from build123d import *

# Parameters (mm, degrees)
F0_W      = 42
F0_H      = 38.608
F1_DEPTH  = 7.493
F2_R      = 1.905
F3_DEPTH  = 7.494
F4_R      = 1.905
F5_DEPTH  = 25.4
F6_R      = 3.302
F6_R_2    = 1.905
F7_DEPTH  = 3.048
F8_R      = 3.5
F9_DEPTH  = 7.494
F10_R     = 12
F11_DEPTH = 3
F13_DEPTH = 3.81


with BuildPart() as f1:
    # F0 (on Top) → F1 (new body)
    with BuildSketch(Plane.XY):
        Rectangle(F0_W, F0_H)
    extrude(amount=F1_DEPTH)

    # F2 (on face) → F3 (cut, through all)
    with BuildSketch(Plane.XY.offset(7.493)):
        with Locations((-14.8492424049, 14.8492424049)):
            Circle(F2_R)
        with Locations((14.8492424049, -14.8492424049)):
            Circle(F2_R)
    extrude(amount=-F3_DEPTH, mode=Mode.SUBTRACT)

    # F4 (on face) → F5 (cut)
    with BuildSketch(Plane.XY.offset(7.493)):
        with Locations((15.5, 15.5)):
            Circle(F4_R)
        with Locations((-15.5, -15.5)):
            Circle(F4_R)
    extrude(amount=-F5_DEPTH, mode=Mode.SUBTRACT)

    # F6 (on face) → F7 (cut)
    with BuildSketch(Plane.XY.offset(7.493)):
        with Locations((15.5, 15.5)):
            Circle(F6_R)
        with Locations((15.5, 15.5)):
            Circle(F6_R_2, mode=Mode.SUBTRACT)
        with Locations((-15.5, -15.5)):
            Circle(F6_R)
        with Locations((-15.5, -15.5)):
            Circle(F6_R_2, mode=Mode.SUBTRACT)
        with Locations((15.5, 15.5)):
            Circle(F6_R_2)
        with Locations((-15.5, -15.5)):
            Circle(F6_R_2)
    extrude(amount=-F7_DEPTH, mode=Mode.SUBTRACT)

    # F8 (on face) → F9 (cut, through all)
    with BuildSketch(Plane.XY.offset(7.493)):
        Circle(F8_R)
    extrude(amount=-F9_DEPTH, mode=Mode.SUBTRACT)

    # F10 (on face) → F11 (cut)
    with BuildSketch(Plane(origin=(0, 0, 0), x_dir=(1, 0, 0), z_dir=(0, 0, -1))):
        Circle(F10_R)
    extrude(amount=-F11_DEPTH, mode=Mode.SUBTRACT)

    # F12 (on face) → F13 (cut)
    with BuildSketch(Plane(origin=(0, 0, 0), x_dir=(1, 0, 0), z_dir=(0, 0, -1))):
        Polygon((18.2782424049, 12.8695083319), (18.2782424049, 16.828976478), (14.8492424049, 18.808710551), (11.4202424049, 16.828976478), (11.4202424049, 12.8695083319), (14.8492424049, 10.8897742588), align=None)
        Polygon((-11.4202424049, -16.828976478), (-11.4202424049, -12.8695083319), (-14.8492424049, -10.8897742588), (-18.2782424049, -12.8695083319), (-18.2782424049, -16.828976478), (-14.8492424049, -18.808710551), align=None)
    extrude(amount=-F13_DEPTH, mode=Mode.SUBTRACT)


solid = f1.part
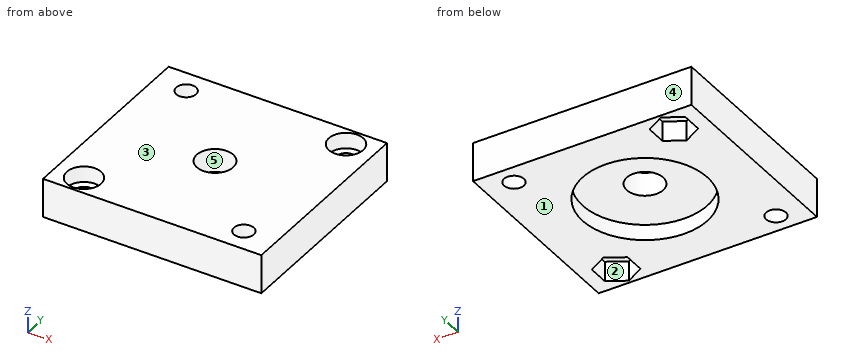
Verification items for the finished model (mm, model axes). Face numbers are marked on the shaded views. A direction names the side the tool comes from. Coordinates: 2 decimals unless noted, no trailing zeros. Write each loop counter-clockwise with the first axis right and the second up, starting at its lowest first coordinate (ties: lowest second). Pieces come first, ordered by that corner, then holes. Notation, with made-up numbers: M -11.5,40 L 20.5,40 A23 ccw 20.5,60 Z; hole C 53,42 d7. An arc over 180 degrees is marked long. Use a Markdown table: item, result.
Q1. Sectioned sample at A-A, the plane x = 0. Record the boundary of the cut face in (y, z), plus the area to 3 significant figures.
Reply:
| item | result |
|---|---|
| outline | M -19.3,0 L -12,0 L -12,3 L -3.5,3 L -3.5,7.49 L -19.3,7.49 Z; M 3.5,3 L 12,3 L 12,0 L 19.3,0 L 19.3,7.49 L 3.5,7.49 Z |
| area | 186 mm² |
Q2. Draft check along Y on the marked faces 3, 4 and 5. Enter one of: +Y half, -Y half, draft (parallel to the pull), parting line (faces both ways), or undercut.
Reply:
| item | result |
|---|---|
| face 3 | draft |
| face 4 | +Y half |
| face 5 | undercut |
Q3. Go/stop test with flat-tipped pins: P1, Ø6.5, axis at x = 0, y = 0, coming from the +Z side; P2, Ø19, axis at x = 0, y = 0, coming from the -Z side; P3, Ø4.5, axis at x = 14.85, y = -14.85, coming from the -Z side. Record where each tip stops, or that it passes through.
Reply:
| item | result |
|---|---|
| P1 | passes through |
| P2 | stops at z = 3 |
| P3 | stops at z = 3.81 |
Q4. Sectioned sample at C-C, the plane z = 5. Record the boundary of the cut face in (x, y) (3 decimals), plus the area to 3 significant figures.
Reply:
| item | result |
|---|---|
| outline | M -21,-19.304 L 21,-19.304 L 21,19.304 L -21,19.304 Z; hole C -15.5,-15.5 d6.604; hole C -14.849,14.849 d3.81; hole C 0,0 d7; hole C 15.5,15.5 d6.604; hole C 14.849,-14.849 d3.81 |
| area | 1,490 mm² |
Q5. Sectioned sample at B-B, the plane y = 0. Record the boundary of the cut face in (x, z).
Reply:
| item | result |
|---|---|
| outline | M -21,0 L -12,0 L -12,3 L -3.5,3 L -3.5,7.49 L -21,7.49 Z; M 3.5,3 L 12,3 L 12,0 L 21,0 L 21,7.49 L 3.5,7.49 Z |
Q6. Set-up check for the marked faces 1 and 2: record each of +Z, -Z, +X, -X, +Y, -Y from which the full face is reachable in a straight line by a thin tool's end or side.
Reply:
| item | result |
|---|---|
| face 1 | -Z, +X, -X, +Y, -Y |
| face 2 | -Z |
Q7. Sectioned sample at D-D, the plane y = -15.5. Record the boundary of the cut face in (x, z) (3 decimals), plus the area to 3 significant figures.
Reply:
| item | result |
|---|---|
| outline | M -21,0 L -17.405,0 L -17.405,4.445 L -18.802,4.445 L -18.802,7.493 L -21,7.493 Z; M -13.595,0 L 11.42,0 L 11.42,3.81 L 13.059,3.81 L 13.059,7.493 L -12.198,7.493 L -12.198,4.445 L -13.595,4.445 Z; M 16.64,3.81 L 18.278,3.81 L 18.278,0 L 21,0 L 21,7.493 L 16.64,7.493 Z |
| area | 238 mm² |
Q8. Thickness scan on line 1 (Y direction, x = 15.5, z = 0.9) (3 decimals); line 2 (Y direction, x = -15.5, z = 1) (3 decimals); line 3 (X direction, y = 13, z = 2.75). Record the ranges inside material, lowest first.
Reply:
| item | result |
|---|---|
| line 1 | y = -19.304 to -18.433, -11.265 to 13.595, 17.405 to 19.304 |
| line 2 | y = -19.304 to -17.405, -13.595 to 11.265, 18.433 to 19.304 |
| line 3 | x = -21 to -18.28, -11.42 to 21 |
